Geometry: see drawing. Coordinates: mm, zero at the bounding-box minimum. Round coordinates to 2 decimals unless told otherwise and drop trailing zeros. Loops run counter-clockwise (first coordinate to the right, second up) from the corner with the lowest first, then second, coordinate; pieces in that order, holes last. Notation, with made-up numbers: (3, 17) - (43, 17) arc R20 ccw to (43, 56) - close; hole circle Ø7 at (72.25, 24.25). An arc over 180 degrees is marked (long way). Write item = value, one per line. Start each with the question number.
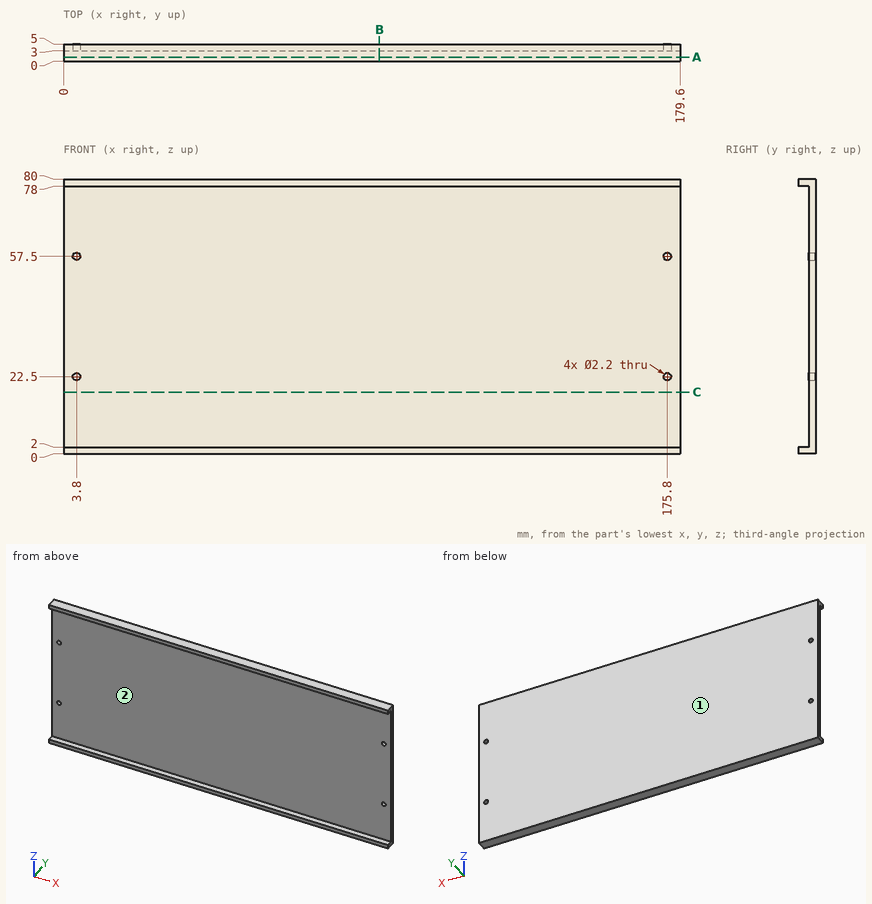
(1) Mould query, pull axis Z, two halves, no side actions, for the marked faces 1 and 2. Classes: +Z half, -Z half, draft (parallel to the pull), parting line (faces both ways), or undercut.
(2) Cut plane C-C (z = 18). Output: boundary loops of the cut face in (x, y).
(3) Material intervals for line 1 along Z through (x, y) = (175.8, 4.2); line 2 along X through (y, z) = (4.2, 57.5); line 3 along Z through (x, y) = (116.5, 0.9), sorted ascending. Write a range as from..to.
(4) Cut plane A-A (y = 1.15). Output: boundary loops of the cut face in (x, z).
(5) Cut plane B-B (x = 92). Output: boundary loops of the cut face in (y, z), and give its area (3 significant figures).
(6) Pin query (flat end, axial travel): P1, Ø3, axis at x = 156, z = 49, coming from the -Y side. Return the tip coordinate at first contact, or that it passes through.
Solution:
q1.face_1 = draft
q1.face_2 = undercut
q2.outline = (0, 3) - (179.6, 3) - (179.6, 5) - (0, 5) - close
q3.line_1 = 0..21.4, 23.6..56.4, 58.6..80
q3.line_2 = 0..2.7, 4.9..174.7, 176.9..179.6
q3.line_3 = 0..2, 78..80
q4.outline = (0, 0) - (179.6, 0) - (179.6, 2) - (0, 2) - close; (0, 78) - (179.6, 78) - (179.6, 80) - (0, 80) - close
q5.outline = (0, 0) - (5, 0) - (5, 80) - (0, 80) - (0, 78) - (3, 78) - (3, 2) - (0, 2) - close
q5.area = 172 mm^2
q6.P1 = 3
